Verification items for this drawing (mm, ordinates from the low corner). A direction names the side the tool comes from. Coordinates: 2 decimals unless noted, no trailing zeros. Order: outer loops, then holes, each group sorted by start corner. A loop starts at its lowest first (then second) coordinate and runs counter-clockwise, first axis right, second up. Notation, with made-up numbers: (73.5, 36.25) - (104.5, 36.25) arc R16 ccw to (104.5, 56.25) - close; hole circle Ø7 at (67.25, -22). An arc over 180 degrees is marked (long way). One line per question, with ' | ' between items. Start each with the question number.
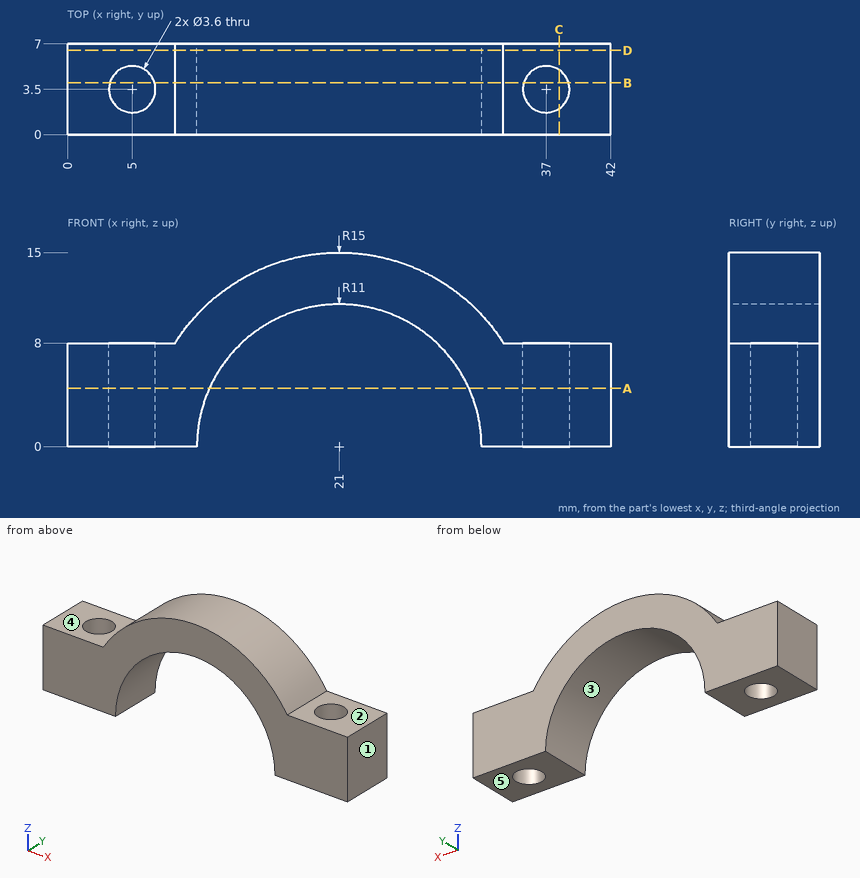
Item 1: Section check B-B (y = 4). Record the cut outline in (x, z).
Item 2: Set-up check for the marked faces 4 and 5: record each of +Z, -Z, +X, -X, +Y, -Y from which the full face is reachable in a straight line by a thin tool's end or side.
Item 3: Gauge pin test, flat ends, axial feed: pin 1 (1.5 mm diameter, centred on x = 16.5, y = 5, fed in from +Z); pin 2 (3 mm diameter, centred on y = 1, z = 11, fed in from -X); pin 3 (3.5 mm diameter, centred on x = 2.5, y = 3, fed in from +Z). Record the tip position at first contact, or that the pin passes through.
Item 4: Thickness scan on probe 1 along Y at (x, z) = (5, 6.25); probe 2 along Z at (x, y) = (38.5, 6.5); probe 3 along X at (y, z) = (3, 6.25). Record the ranges inside material, lowest first. Write a range as from..to.
Item 5: Section check C-C (x = 38). Record the cut outline in (y, z).
Item 6: Mould release check, pull along X, two halves, no side actions. Record for the marked faces 1, 2 and 3: +X half, -X half, draft (parallel to the pull), parting line (faces both ways), or undercut.
Item 7: Section check A-A (z = 4.5). Record the cut outline in (x, y).
Item 8: Section check D-D (y = 6.5). Record the cut outline in (x, z), then the cut area to 3 significant figures.
Completed:
1) outline: (0, 0) - (3.27, 0) - (3.27, 8) - (0, 8) - close; (6.73, 0) - (10, 0) arc R11 cw to (32, 0) - (35.27, 0) - (35.27, 8) - (33.69, 8) arc R15 ccw to (8.31, 8) - (6.73, 8) - close; (38.73, 0) - (42, 0) - (42, 8) - (38.73, 8) - close
2) face 4: +Z, -X, +Y, -Y | face 5: -Z, +X, -X, +Y, -Y
3) pin 1: stops at z = 14.52 | pin 2: stops at x = 9.39 | pin 3: stops at z = 8
4) probe 1: y = 0..1.7, 5.3..7 | probe 2: z = 0..8 | probe 3: x = 0..3.27, 6.73..11.95, 30.05..35.27, 38.73..42
5) outline: (0, 0) - (2, 0) - (2, 8) - (0, 8) - close; (5, 0) - (7, 0) - (7, 8) - (5, 8) - close
6) face 1: +X half | face 2: draft | face 3: undercut
7) outline: (0, 0) - (10.96, 0) - (10.96, 7) - (0, 7) - close; (31.04, 0) - (42, 0) - (42, 7) - (31.04, 7) - close; hole circle Ø3.6 at (5, 3.5); hole circle Ø3.6 at (37, 3.5)
8) outline: (0, 0) - (10, 0) arc R11 cw to (32, 0) - (42, 0) - (42, 8) - (33.69, 8) arc R15 ccw to (8.31, 8) - (0, 8) - close | area: 271 mm^2
